The model under review builds one solid part; all positions refer to its coordinate system, in mm. A direction names the side the tool comes from. Coordinates: 2 decimals unless noted, no trailing zeros. Loops run counter-clockwise (first coordinate to the right, second up) from the corner with the lowest first, then second, coordinate; pieces in that order, holes last. Notation, with made-up numbers: M 30.25,-19.75 L 51.25,-19.75 A9 cw 51.25,-11.75 Z; hole C 51.25,-21 d8. An arc over 180 degrees is marked long. Return JSON: item names as keys, results as strings.
```python
from build123d import *

# Parameters (mm, degrees)
SKETCH1_R           = 2.032
SKETCH1_W           = 6.35
SKETCH1_H           = 6.35
BOSS_EXTRUDE2_DEPTH = 6.35
CUT_EXTRUDE1_START  = -6.35
SKETCH3_R           = 3.175
CUT_EXTRUDE1_DEPTH  = 195.131829617


with BuildPart() as part:
    # Sketch1 → Boss-Extrude2 (new body)
    with BuildSketch(Plane.XY):
        with BuildLine():
            Line((21.7678, 129.667339502), (0, 129.667339502))
            Line((0, 129.667339502), (0, 109.016949915))
            ThreePointArc((0, 109.016949915), (-0.215035851, 107.994139226), (-0.823733627, 107.1445104))
            Line((-0.823733627, 107.1445104), (-118.042304389, -0.297300013))
            ThreePointArc((-118.042304389, -0.297300013), (-118.837809221, -0.792094788), (-119.758570763, -0.964860498))
            Line((-119.758570763, -0.964860498), (-135.676357929, -0.964860498))
            Line((-135.676357929, -0.964860498), (-135.676357929, -29.082660498))
            Line((-135.676357929, -29.082660498), (-97.576357929, -29.082660498))
            Line((-97.576357929, -29.082660498), (-97.576357929, -22.732660498))
            Line((-97.576357929, -22.732660498), (-46.776357929, -22.732660498))
            Line((-46.776357929, -22.732660498), (-46.776357929, -29.082660498))
            Line((-46.776357929, -29.082660498), (-8.676357929, -29.082660498))
            Line((-8.676357929, -29.082660498), (-8.676357929, -22.732660498))
            Line((-8.676357929, -22.732660498), (42.123642071, -22.732660498))
            Line((42.123642071, -22.732660498), (42.123642071, -29.082660498))
            Line((42.123642071, -29.082660498), (80.223642071, -29.082660498))
            Line((80.223642071, -29.082660498), (80.223642071, 0))
            Line((80.223642071, 0), (22.314225969, 73.349225433))
            ThreePointArc((22.314225969, 73.349225433), (21.908291921, 74.090114432), (21.7678, 74.923157637))
            Line((21.7678, 74.923157637), (21.7678, 129.667339502))
        make_face()
        with Locations((-116.626357929, -25.907660498)):
            Circle(SKETCH1_R, mode=Mode.SUBTRACT)
        with Locations((-27.726357929, -25.907660498)):
            Circle(SKETCH1_R, mode=Mode.SUBTRACT)
        with Locations((61.173642071, -25.907660498)):
            Circle(SKETCH1_R, mode=Mode.SUBTRACT)
        with Locations((10.8839, 107.442339502)):
            Circle(SKETCH1_R, mode=Mode.SUBTRACT)
        with BuildLine():
            Line((24.3078, 0), (52.822865129, 0))
            ThreePointArc((52.822865129, 0), (55.108624062, 1.432342065), (54.81643916, 4.113932204))
            Line((54.81643916, 4.113932204), (26.301374031, 40.231684398))
            ThreePointArc((26.301374031, 40.231684398), (23.474756795, 41.057260272), (21.7678, 38.657752193))
            Line((21.7678, 38.657752193), (21.7678, 2.54))
            ThreePointArc((21.7678, 2.54), (22.511748776, 0.743948776), (24.3078, 0))
        make_face(mode=Mode.SUBTRACT)
        with BuildLine():
            Line((0, 2.54), (0, 74.05849329))
            ThreePointArc((0, 74.05849329), (-1.517189311, 76.38345744), (-4.256266373, 75.930932805))
            Line((-4.256266373, 75.930932805), (-82.28264674, 4.412439515))
            ThreePointArc((-82.28264674, 4.412439515), (-82.933614657, 1.619238458), (-80.566380367, 0))
            Line((-80.566380367, 0), (-2.54, 0))
            ThreePointArc((-2.54, 0), (-0.743948776, 0.743948776), (0, 2.54))
        make_face(mode=Mode.SUBTRACT)
        with Locations((10.8839, 116.967339502)):
            Rectangle(SKETCH1_W, SKETCH1_H, mode=Mode.SUBTRACT)
        with Locations((10.8839, 97.917339502)):
            Rectangle(SKETCH1_W, SKETCH1_H, mode=Mode.SUBTRACT)
    extrude(amount=BOSS_EXTRUDE2_DEPTH)

    # Sketch3 → Cut-Extrude1 (cut, through all)
    with BuildSketch(Plane.XY.offset(6.35).offset(CUT_EXTRUDE1_START)):
        with Locations((10.8839, -10.16)):
            Circle(SKETCH3_R)
        with Locations((31.2039, -10.16)):
            Circle(SKETCH3_R)
        with Locations((51.5239, -10.16)):
            Circle(SKETCH3_R)
        with Locations((71.8439, -10.16)):
            Circle(SKETCH3_R)
    extrude(amount=CUT_EXTRUDE1_DEPTH, mode=Mode.SUBTRACT)


solid = part.part
```
1. Machinability: for faces 4 (the face through (42.124, -26, 3)), 5 (the face through (-128, -0.965, 3)), 6 (the face through (61, -29.083, 3)), 7 (the face through (11, 120.142, 3)), which of the approach directions +Z, -Z, +X, -X, +Y, -Y give a long, thin tool a straight path to every point of the face, cutting with its end or side? Answer none if there is none.
Check values:
{"face 4": "+Z, -Z, -Y", "face 5": "+Z, -Z, -X, +Y", "face 6": "+Z, -Z, +X, -X, -Y", "face 7": "+Z, -Z"}
2. Add section D-D on x = 3.5. Give the boundary of the cut face in (y, z).
Check values:
{"outline": "M -22.73,0 L 129.67,0 L 129.67,6.35 L -22.73,6.35 Z"}
3. Insertion check: pin 1 Ø2 at (y, z) = (20.5, 2) entering from -X; pin 2 Ø3 at (y, z) = (98, 3.5) entering from +X; pin 3 Ø1.5 at (x, z) = (26, 2.5) entering from -Y. Each pin has a flat end and moves straight along its axis. Give the tip position at first contact, or say it passes through.
Check values:
{"pin 1": "x = -96.44", "pin 2": "x = 21.77", "pin 3": "y = -22.73"}
4. The part is to be moulded in two halves that separate along X. For faces 1 (the face through (51.674, 36.161, 3.131)), 2 (the face through (7.709, 98, 3)), 3 (the face through (-28, -29.083, 3)), say which applies: released by +X, released by -X, zero draft, split by the parting line, or undercut.
Check values:
{"face 1": "released by +X", "face 2": "undercut", "face 3": "zero draft"}
5. To check wall thickness, follow line 1 (X direction, y = -10.16, z = 3.75); line 2 (X direction, y = 40.5, z = 0.75); line 3 (X direction, y = 17.5, z = 1.25). State the ranges of each line that lie inside material, in increasing order.
Check values:
{"line 1": "-135.68 to 7.71, 14.06 to 28.03, 34.38 to 48.35, 54.7 to 68.67, 75.02 to 80.22", "line 2": "-73.53 to -42.91, 0 to 22.56, 26.06 to 48.25", "line 3": "-98.63 to -68, 0 to 21.77, 44.25 to 66.41"}
6. Add section B-B on y = 9. Give the boundary of the cut face in (x, z).
Check values:
{"outline": "M -107.9,0 L -77.28,0 L -77.28,6.35 L -107.9,6.35 Z; M 0,0 L 21.77,0 L 21.77,6.35 L 0,6.35 Z; M 50.96,0 L 73.12,0 L 73.12,6.35 L 50.96,6.35 Z"}
7. Add section C-C on z = 3.5. State how many separate pieces and enclosed holes the cut face has, plus the area to 3 significant figures.
Check values:
{"separate pieces": "1", "enclosed holes": "12", "area": "12,400 mm²"}
8. Add section A-A on y = -10.16. Give the boundary of the cut face in (x, z).
Check values:
{"outline": "M -135.68,0 L 7.71,0 L 7.71,6.35 L -135.68,6.35 Z; M 14.06,0 L 28.03,0 L 28.03,6.35 L 14.06,6.35 Z; M 34.38,0 L 48.35,0 L 48.35,6.35 L 34.38,6.35 Z; M 54.7,0 L 68.67,0 L 68.67,6.35 L 54.7,6.35 Z; M 75.02,0 L 80.22,0 L 80.22,6.35 L 75.02,6.35 Z"}
